from build123d import *

# Parameters (mm, degrees)
SKETCH1_W           = 50
SKETCH1_H           = 60
SKETCH1_R           = 2.5
SKETCH1_W_2         = 20
SKETCH1_H_2         = 40
BOSS_EXTRUDE1_DEPTH = 5


with BuildPart() as part:
    # Sketch1 → Boss-Extrude1 (new body)
    with BuildSketch(Plane(origin=(0, 0, 0), x_dir=(1, 0, 0), z_dir=(0, 1, 0))):
        with Locations((-25.619469027, 11.991150442)):
            Rectangle(SKETCH1_W, SKETCH1_H)
        with Locations(Location((-10.619469027, 31.991150442, 0), (0, 0, 270))):
            Circle(SKETCH1_R, mode=Mode.SUBTRACT)
        with Locations(Location((-10.619469027, -8.008849558, 0), (0, 0, 90))):
            Circle(SKETCH1_R, mode=Mode.SUBTRACT)
        with Locations(Location((-43.119469027, 35.991150442, 0), (0, 0, 270))):
            Circle(SKETCH1_R, mode=Mode.SUBTRACT)
        with Locations(Location((-33.119469027, 35.991150442, 0), (0, 0, 270))):
            Circle(SKETCH1_R, mode=Mode.SUBTRACT)
        with Locations(Location((-43.119469027, -12.008849558, 0), (0, 0, 90))):
            Circle(SKETCH1_R, mode=Mode.SUBTRACT)
        with Locations(Location((-33.119469027, -12.008849558, 0), (0, 0, 90))):
            Circle(SKETCH1_R, mode=Mode.SUBTRACT)
        with Locations((-38.119469027, 11.991150442)):
            Rectangle(SKETCH1_W_2, SKETCH1_H_2, mode=Mode.SUBTRACT)
    extrude(amount=BOSS_EXTRUDE1_DEPTH)


solid = part.part
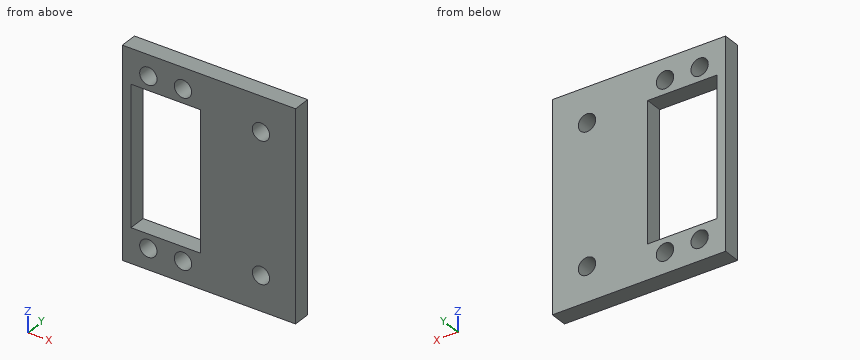
The listing builds one solid part. Answer for the finished solid, in the listing's coordinates (mm). Round coordinates to 2 decimals unless told otherwise and drop trailing zeros. Order: outer loops, then holes, each group sorted by start corner. A loop starts at its lowest first (then second) coordinate and runs counter-clockwise, first axis right, second up. Notation, with made-up numbers: (15.25, 25) -> (73.25, 25) arc R16 cw to (73.25, 32) -> close; hole circle Ø9 at (73.5, 43). An arc over 180 degrees is marked (long way). Write each question's results on one line, items separated by ' | '. Start each with the question number.
Q1. Find section C-C (y = 3.05). Determine the outline of the cut face in (x, z).
Q2. Straight lines are drawn through the part: probe 1 along X at (y, z) = (4.1, -4); probe 2 along Z at (x, y) = (-33, 2.75); probe 3 along X at (y, z) = (0.55, -30). For each, find the intervals that lie inside material, in ascending order. Write a range as from..to.
Q3. Find section A-A (x = -47). Determine the outline of the cut face in (y, z), then the cut area to 3 significant figures.
Q4. Find section B-B (z = -7). Determine the outline of the cut face in (x, y), then the cut area to 3 significant figures.
Q5. This flat-tipped pin is pushed along its axis until it touches: pin 1 (4.5 mm diameter, centred on x = -33.12, z = -35.99, fed in from +Y). Where does it stop, or does it pass through?
Worked answers:
1) outline: (-50.62, -41.99) -> (-0.62, -41.99) -> (-0.62, 18.01) -> (-50.62, 18.01) -> close; hole (-48.12, -31.99) -> (-28.12, -31.99) -> (-28.12, 8.01) -> (-48.12, 8.01) -> close; hole circle Ø5 at (-43.12, -35.99); hole circle Ø5 at (-43.12, 12.01); hole circle Ø5 at (-33.12, -35.99); hole circle Ø5 at (-33.12, 12.01); hole circle Ø5 at (-10.62, -31.99); hole circle Ø5 at (-10.62, 8.01)
2) probe 1: x = -50.62..-48.12, -28.12..-0.62 | probe 2: z = -41.99..-38.49, -33.49..-31.99, 8.01..9.51, 14.51..18.01 | probe 3: x = -50.62..-48.12, -28.12..-12.13, -9.11..-0.62
3) outline: (0, -41.99) -> (5, -41.99) -> (5, -31.99) -> (0, -31.99) -> close; (0, 8.01) -> (5, 8.01) -> (5, 18.01) -> (0, 18.01) -> close | area: 100 mm2
4) outline: (-50.62, 0) -> (-48.12, 0) -> (-48.12, 5) -> (-50.62, 5) -> close; (-28.12, 0) -> (-0.62, 0) -> (-0.62, 5) -> (-28.12, 5) -> close | area: 150 mm2
5) pin 1: passes through
